Check sheet for the modelled part. Datum: model origin and axes. Units: mm. A direction names the side the tool comes from. Give positions to 0.01 mm unless a question says otherwise; leave off trailing zeros. Order: outer loops, then holes, each group sorted by start corner. A loop starts at its lowest first (then second) coordinate and runs counter-clockwise, first axis right, second up.
Item 1: Access from +Z, -Z, +X, -X, +Y, -Y to the whole of each face (thin tool, end or side, straight path). Record for faces 1 (the flat face through (84, 50, 2)), 2 (the flat face through (127, 42.5, 3)).
Item 2: Gauge pin test, flat ends, axial feed: P1, Ø8, axis at x = 75.5, y = 19.5, coming from the +Z side; P2, Ø1.5, axis at y = 22, z = 3.5, coming from the +X side; P3, Ø0.8, axis at x = 70, z = 3.5, coming from the -Y side. Record the tip position at first contact, or that the pin passes through.
Item 3: Sectioned sample at B-B on z = 1.2. Count the separate pieces of the cut face and the enclosed holes in it, and give its area (3 significant figures).
Item 4: Sectioned sample at A-A on x = 70. Record the boundary of the cut face in (y, z).
Item 5: Material ranges on line 1 along Y through (x, z) = (77.5, 1.2); line 2 along Z through (x, y) = (134.5, 36.5); line 3 along Y through (x, z) = (104, 3.7), recorded low to high.
Item 6: Release check for a two-part mould opening along X. For faces 3 (the flat face through (75, 45, 3)), 4 (the flat face through (84, 25, 0)), 5 (the flat face through (25, 42.5, 3)) record: released by +X, released by -X, zero draft, split by the parting line, or undercut.
Item 7: Sectioned sample at C-C on y = 17. Record the boundary of the cut face in (x, z).
from build123d import *

# Parameters (mm, degrees)
SKETCH_W        = 170
SKETCH_H        = 50
PAD_DEPTH       = 5
SKETCH001_W     = 170
SKETCH001_H     = 40
POCKET_DEPTH    = 2
FILLET_R        = 1
SKETCH002_W     = 3
SKETCH002_H     = 5
POCKET001_DEPTH = 5.001
FILLET001_R     = 0.3
FILLET002_R     = 0.3


with BuildPart() as part:
    # Sketch → Pad (new body)
    with BuildSketch(Plane.XY):
        with Locations((85, 25)):
            Rectangle(SKETCH_W, SKETCH_H)
    extrude(amount=PAD_DEPTH)

    # Sketch001 (on Face6 of Pad) → Pocket (cut)
    with BuildSketch(Plane.XY.offset(5)):
        with Locations((85, 20)):
            Rectangle(SKETCH001_W, SKETCH001_H)
    extrude(amount=-POCKET_DEPTH, mode=Mode.SUBTRACT)

    # Fillet
    fillet_edges = [part.edges().sort_by_distance(p)[0] for p in [
        (0, 20, 3),
        (85, 0, 3),
        (170, 20, 3),
        (85, 40, 5),
        (170, 45, 5),
        (85, 50, 5),
        (0, 45, 5),
        (0, 40, 4),
        (170, 40, 4),
    ]]
    fillet(fillet_edges, radius=FILLET_R)

    # Sketch002 (on Face10 of Fillet) → Pocket001 (cut, through all)
    with BuildSketch(Plane.XY.offset(5)):
        with Locations((8.5, 45)):
            Rectangle(SKETCH002_W, SKETCH002_H)
        with Locations((25.5, 45)):
            Rectangle(SKETCH002_W, SKETCH002_H)
        with Locations((42.5, 45)):
            Rectangle(SKETCH002_W, SKETCH002_H)
        with Locations((161.5, 45)):
            Rectangle(SKETCH002_W, SKETCH002_H)
        with Locations((59.5, 45)):
            Rectangle(SKETCH002_W, SKETCH002_H)
        with Locations((76.5, 45)):
            Rectangle(SKETCH002_W, SKETCH002_H)
        with Locations((93.5, 45)):
            Rectangle(SKETCH002_W, SKETCH002_H)
        with Locations((110.5, 45)):
            Rectangle(SKETCH002_W, SKETCH002_H)
        with Locations((127.5, 45)):
            Rectangle(SKETCH002_W, SKETCH002_H)
        with Locations((144.5, 45)):
            Rectangle(SKETCH002_W, SKETCH002_H)
    extrude(amount=-POCKET001_DEPTH, mode=Mode.SUBTRACT)

    # Fillet001
    fillet001_edges = [part.edges().sort_by_distance(p)[0] for p in [
        (10, 45, 5),
        (8.5, 42.5, 5),
        (7, 45, 5),
        (8.5, 47.5, 5),
        (25.5, 47.5, 5),
        (24, 45, 5),
        (25.5, 42.5, 5),
        (27, 45, 5),
        (41, 45, 5),
        (42.5, 47.5, 5),
        (44, 45, 5),
        (42.5, 42.5, 5),
        (59.5, 47.5, 5),
        (58, 45, 5),
        (61, 45, 5),
        (59.5, 42.5, 5),
        (76.5, 47.5, 5),
        (75, 45, 5),
        (76.5, 42.5, 5),
        (78, 45, 5),
        (92, 45, 5),
        (93.5, 47.5, 5),
        (95, 45, 5),
        (93.5, 42.5, 5),
        (110.5, 47.5, 5),
        (109, 45, 5),
        (112, 45, 5),
        (110.5, 42.5, 5),
        (127.5, 47.5, 5),
        (126, 45, 5),
        (129, 45, 5),
        (127.5, 42.5, 5),
        (143, 45, 5),
        (144.5, 47.5, 5),
        (146, 45, 5),
        (144.5, 42.5, 5),
        (161.5, 47.5, 5),
        (160, 45, 5),
        (163, 45, 5),
        (161.5, 42.5, 5),
    ]]
    fillet(fillet001_edges, radius=FILLET001_R)

    # Fillet002
    fillet002_edges = [part.edges().sort_by_distance(p)[0] for p in [
        (7, 45, 0),
        (8.5, 42.5, 0),
        (10, 45, 0),
        (8.5, 47.5, 0),
        (25.5, 42.5, 0),
        (24, 45, 0),
        (25.5, 47.5, 0),
        (27, 45, 0),
        (42.5, 42.5, 0),
        (41, 45, 0),
        (44, 45, 0),
        (42.5, 47.5, 0),
        (58, 45, 0),
        (59.5, 42.5, 0),
        (61, 45, 0),
        (59.5, 47.5, 0),
        (76.5, 42.5, 0),
        (75, 45, 0),
        (76.5, 47.5, 0),
        (78, 45, 0),
        (92, 45, 0),
        (93.5, 42.5, 0),
        (95, 45, 0),
        (93.5, 47.5, 0),
        (110.5, 42.5, 0),
        (109, 45, 0),
        (110.5, 47.5, 0),
        (112, 45, 0),
        (127.5, 42.5, 0),
        (126, 45, 0),
        (127.5, 47.5, 0),
        (129, 45, 0),
        (143, 45, 0),
        (144.5, 42.5, 0),
        (146, 45, 0),
        (144.5, 47.5, 0),
        (161.5, 42.5, 0),
        (160, 45, 0),
        (163, 45, 0),
        (161.5, 47.5, 0),
    ]]
    fillet(fillet002_edges, radius=FILLET002_R)


solid = part.part
Report:
1. face 1: +Z, -Z, +X, -X, +Y
1. face 2: +Z, -Z
2. P1: stops at z = 3
2. P2: stops at x = 169.66
2. P3: stops at y = 40
3. separate pieces: 1
3. enclosed holes: 10
3. area: 8,350 mm2
4. outline: (0, 0) - (50, 0) - (50, 4) arc R1 ccw to (49, 5) - (41, 5) arc R1 ccw to (40, 4) - (40, 3) - (1, 3) arc R1 ccw to (0, 2) - close
5. line 1: y = 0 to 42.5, 47.5 to 50
5. line 2: z = 0 to 3
5. line 3: y = 40 to 50
6. face 3: undercut
6. face 4: zero draft
6. face 5: undercut
7. outline: (0, 0) - (170, 0) - (170, 2) arc R1 ccw to (169, 3) - (1, 3) arc R1 ccw to (0, 2) - close
